```python
from build123d import *

# Parameters (mm, degrees)
SWEEP1_DEPTH        = 5
CIRPATTERN1_COUNT   = 4
SKETCH1_R           = 10
SKETCH1_R_2         = 9.6
SKETCH1_R_3         = 3
SKETCH1_R_4         = 1.5
BOSS_EXTRUDE1_DEPTH = 5
CUT_EXTRUDE1_DEPTH  = 5


# Read off the part's stored shape, not the designer's step: Sweep1
with BuildPart() as part:
    # Sweep1 outline → Sweep1 (new body)
    with BuildSketch(Plane(origin=(0, 0, 0), x_dir=(1, 0, 0), z_dir=(0, 1, 0))):
        with BuildLine():
            add(Edge.make_bspline(
                [(-9.997767253, 0.042204416), (-9.893548222, 1.024445624), (-9.643855436, 1.975253332), (-8.514500953, 4.619730854), (-7.250148261, 6.089394307), (-4.220454712, 8.034217024), (-2.465869735, 8.506161552), (0.899525972, 8.415541149), (2.500050194, 7.856354951), (5.039536559, 6.020831642), (5.972232345, 4.75284276), (6.951327861, 2.022470319), (6.997401809, 0.570143689), (6.315351727, -2.009640106), (5.592555924, -3.128989147), (3.739249202, -4.711480962), (2.61745741, -5.171210965), (0.421238612, -5.385789198), (-0.6444086, -5.14284378), (-2.363661266, -4.165013808), (-3.011596763, -3.436835308), (-3.744471685, -1.846203068), (-3.828769264, -0.992292459), (-3.523310038, 0.505264712), (-3.138015362, 1.141752965), (-2.151370993, 2.005668845), (-1.557863942, 2.230032974), (-0.453404495, 2.27341979), (0.04937349, 2.094819441), (0.756807528, 1.505326697), (0.956441656, 1.101049011), (0.984935122, 0.319516548), (0.808711828, -0.048952614), (0.355558233, -0.346460579), (0.179752495, -0.399999938), (0, -0.4)],
                knots=[0, 0, 0, 0, 0.03125, 0.03125, 0.09375, 0.09375, 0.15625, 0.15625, 0.21875, 0.21875, 0.28125, 0.28125, 0.34375, 0.34375, 0.40625, 0.40625, 0.46875, 0.46875, 0.53125, 0.53125, 0.59375, 0.59375, 0.65625, 0.65625, 0.71875, 0.71875, 0.78125, 0.78125, 0.84375, 0.84375, 0.90625, 0.90625, 0.96875, 0.96875, 1, 1, 1, 1], degree=3))
            Line((-9.997767253, 0.042204416), (-9.6, 0))
            add(Edge.make_bspline(
                [(-9.6, 0), (-9.500000002, 0.942477768), (-9.260276395, 1.854965201), (-8.178082578, 4.389012093), (-6.966588285, 5.79609643), (-4.07185486, 7.654285459), (-2.396315093, 8.104143661), (0.80843742, 8.017848911), (2.331018658, 7.48498264), (4.739932394, 5.743836325), (5.622987086, 4.541754089), (6.547526362, 1.963520879), (6.589948056, 0.593934112), (5.949379501, -1.82895008), (5.270769692, -2.877772985), (3.541549476, -4.354310455), (2.496772138, -4.781097682), (0.46413157, -4.979693743), (-0.518811459, -4.754107144), (-2.093750636, -3.858355877), (-2.683547792, -3.192955292), (-3.345933745, -1.755312325), (-3.419635874, -0.987893302), (-3.148583322, 0.340980176), (-2.807479524, 0.899505485), (-1.954895304, 1.646036894), (-1.447858478, 1.834045854), (-0.532007817, 1.870023456), (-0.1264769, 1.720682196), (0.420528321, 1.264871984), (0.561230213, 0.962417719), (0.580677698, 0.429001097), (0.461370534, 0.201510606), (0.199937884, 0.029872802), (0.099999829, 1.9e-08), (0, 0)],
                knots=[0, 0, 0, 0, 0.03125, 0.03125, 0.09375, 0.09375, 0.15625, 0.15625, 0.21875, 0.21875, 0.28125, 0.28125, 0.34375, 0.34375, 0.40625, 0.40625, 0.46875, 0.46875, 0.53125, 0.53125, 0.59375, 0.59375, 0.65625, 0.65625, 0.71875, 0.71875, 0.78125, 0.78125, 0.84375, 0.84375, 0.90625, 0.90625, 0.96875, 0.96875, 1, 1, 1, 1], degree=3))
            Line((0, 0), (0, -0.4))
        make_face()
    sweep1 = extrude(amount=SWEEP1_DEPTH)

    # CirPattern1: Sweep1 ×4 about axis
    cirpattern1_axis = Axis((0, 0, 0), (0, 1, 0))
    for i in range(1, CIRPATTERN1_COUNT):
        add(sweep1.rotate(cirpattern1_axis, i * 360 / CIRPATTERN1_COUNT))

    # Sketch1 → Boss-Extrude1 (add)
    # profile 1 of 3: a face of its own
    with BuildSketch(Plane(origin=(0, 0, 0), x_dir=(1, 0, 0), z_dir=(0, 1, 0))):
        with Locations(Location((0, 0, 0), (0, 0, 270))):
            Circle(SKETCH1_R)
        Circle(SKETCH1_R_2, mode=Mode.SUBTRACT)
    # profile 2 of 3: a face of its own
    with BuildSketch(Plane(origin=(0, 0, 0), x_dir=(1, 0, 0), z_dir=(0, 1, 0))):
        Circle(SKETCH1_R_3)
        Circle(SKETCH1_R_4, mode=Mode.SUBTRACT)
    # profile 3 of 3: a face of its own
    with BuildSketch(Plane(origin=(0, 0, 0), x_dir=(1, 0, 0), z_dir=(0, 1, 0))):
        with BuildLine():
            Line((-1, 0), (-1, 1.118033989))
            ThreePointArc((-1, 1.118033989), (-1.5, 0), (-1, -1.118033989))
            Line((-1, -1.118033989), (-1, 0))
        make_face()
    extrude(amount=BOSS_EXTRUDE1_DEPTH)

    # Sketch1<3> → Cut-Extrude1 (cut)
    with BuildSketch(Plane(origin=(0, 0, 0), x_dir=(1, 0, 0), z_dir=(0, 1, 0))):
        with BuildLine():
            ThreePointArc((1.5, 0), (0.612372436, 1.369306394), (-1, 1.118033989))
            Line((-1, 1.118033989), (-1, 0))
            Line((-1, 0), (-1, -1.118033989))
            ThreePointArc((-1, -1.118033989), (0.612372436, -1.369306394), (1.5, 0))
        make_face()
    extrude(amount=CUT_EXTRUDE1_DEPTH, mode=Mode.SUBTRACT)


solid = part.part
```
Model file for the job. Use its own axes, mm. A direction names the side the tool comes from. Round coordinates to 2 decimals unless told otherwise and drop trailing zeros. Put each result on its own line as item: value.
Item 1: Tool access for faces 1 (the flat face through (2, 5, 0)), 2 (the flat face through (-1, 2, 0)): list every direction of +Z, -Z, +X, -X, +Y, -Y with a clear straight run to the whole face (end or side of a thin tool).
Responses:
face 1: +Z, -Z, +X, -X, +Y
face 2: +Y, -Y
Item 2: Cut at A-A (z = 4). State how many separate pieces and enclosed holes the cut face has, and give its area (3 significant figures).
Responses:
separate pieces: 9
enclosed holes: 0
area: 22.5 mm²
Item 3: Flat gauge pins, fed straight in: P1, Ø3, axis at x = 6, z = 6, coming from the +Y side; P2, Ø1, axis at y = 2.5, z = -3, coming from the +X side; P3, Ø2, axis at x = 2, y = 2.5, coming from the -Z side. Where does each tip first touch, or does it go through?
Responses:
P1: y = 5
P2: x = 9.68
P3: z = -9.95
Item 4: Probe L1, parallel to Z at x = 8.5, y = 4.75; L2, parallel to Z at x = -7, y = 3.4. List the from-to ranges inside material, lowest first. Write a range as from..to.
Responses:
L1: -5.27..-4.46, 3.52..4.3, 4.46..5.27
L2: -7.14..-6.57, -6.08..-5.52, -3.68..-2.94, 5.06..5.83, 6.57..7.14
Item 5: Mould opens along Z. For faces 3 (the cylindrical face through (-9.76, 2.46, -2.17)), 4 (the flat face through (2, 0, 0)), 5 (the cylindrical face through (1.093, 2.465, 2.794)), 6 (the cylindrical face through (-8.03, 2.46, 5.26)) say: +Z half, -Z half, draft (parallel to the pull), parting line (faces both ways), or undercut.
Responses:
face 3: parting line
face 4: draft
face 5: undercut
face 6: undercut
